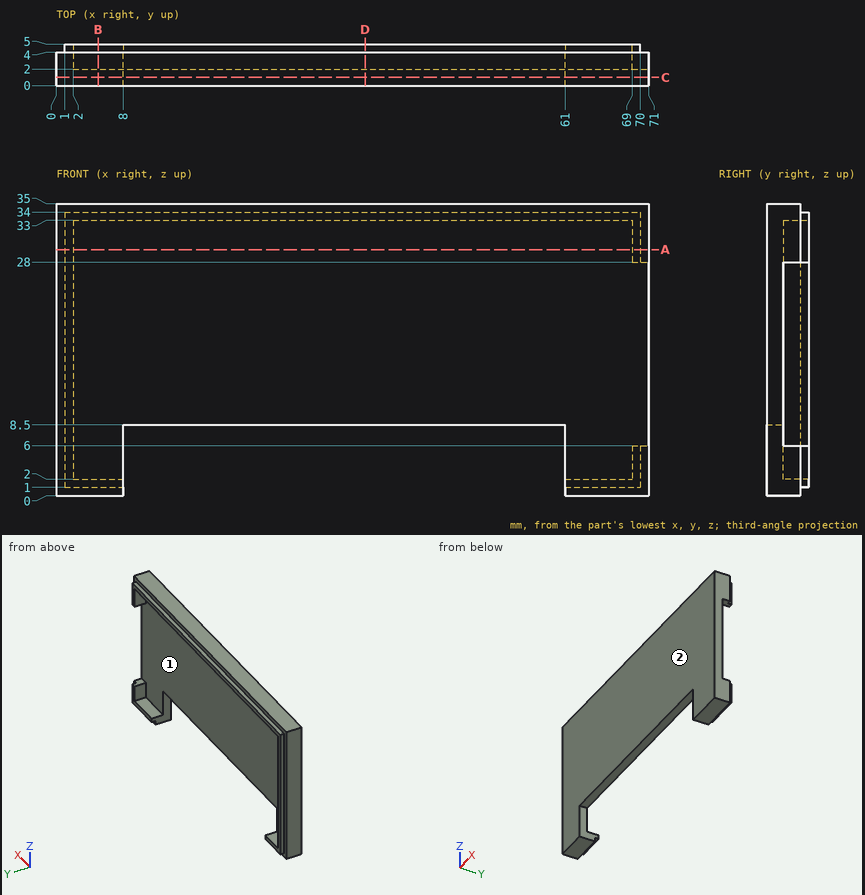
Check sheet for the drawn part. Datum: minimum x, y, z corner. Units: mm. Give positions to 0.01 mm unless a question says otherwise; leave off trailing zeros. Write each loop counter-clockwise with the first axis right and the second up, starting at its lowest first coordinate (ties: lowest second). Pieces come first, ordered by that corner, then holes. Notation, with made-up numbers: (48, -19.75) -> (52, -19.75) arc R22 cw to (52, 8.25) -> close; hole circle Ø2 at (-25, 6.5). An arc over 180 degrees is marked (long way). Use one line per item in the form item = value. Start each with the question number.
1. Section check A-A (z = 29.5). Record the cut outline in (x, y), and give its area (3 significant figures).
2. Section check B-B (x = 5). Record the cut outline in (y, z).
3. Section check C-C (y = 1). Record the cut outline in (x, z), and give its area (3 significant figures).
4. Mould release check, pull along Z, two halves, no side actions. Record for the marked faces 1 and 2: pulls with the +Z half, pulls with the -Z half, needs draft (parallel to the pull), parting line crosses it, or undercut.
5. Go/stop test with flat-tipped pins: P1, Ø0.8, axis at y = 4.5, z = 3.5, coming from the +X side; P2, Ø4, axis at x = 63.5, z = 12.5, coming from the -Y side; P3, Ø1.8, axis at x = 68, z = 4.5, coming from the +Y side; P4, Ø2, axis at x = 11.5, y = 1, coming from the -Z side. Record where each tip stops, or that it passes through.
6. Section check D-D (x = 37). Record the cut outline in (y, z), and give its area (3 significant figures).
7. Thickness scan on line 1 along Z through (x, y) = (4, 3.4); line 2 along X through (y, z) = (1.8, 8); line 3 along X through (y, z) = (4.45, 29.5). Record the ranges inside material, lowest first. Write a range as from..to.
Conclusion:
q1.outline = (0, 0) -> (71, 0) -> (71, 4) -> (70, 4) -> (70, 5) -> (69, 5) -> (69, 2) -> (2, 2) -> (2, 5) -> (1, 5) -> (1, 4) -> (0, 4) -> close
q1.area = 152 mm²
q2.outline = (0, 0) -> (4, 0) -> (4, 1) -> (5, 1) -> (5, 2) -> (2, 2) -> (2, 33) -> (5, 33) -> (5, 34) -> (4, 34) -> (4, 35) -> (0, 35) -> close
q3.outline = (0, 0) -> (8, 0) -> (8, 8.5) -> (61, 8.5) -> (61, 0) -> (71, 0) -> (71, 35) -> (0, 35) -> close
q3.area = 2,030 mm²
q4.face_1 = undercut
q4.face_2 = needs draft
q5.P1 = 70
q5.P2 = 0
q5.P3 = 2
q5.P4 = 8.5
q6.outline = (0, 8.5) -> (2, 8.5) -> (2, 33) -> (5, 33) -> (5, 34) -> (4, 34) -> (4, 35) -> (0, 35) -> close
q6.area = 58.0 mm²
q7.line_1 = 0..2, 33..35
q7.line_2 = 0..8, 61..71
q7.line_3 = 1..2, 69..70
